Here's how the part is built. I have some questions about the finished solid (model axes, mm). Face numbers are marked on the shaded views. A direction names the side the tool comes from. Round coordinates to 2 decimals unless told otherwise and drop trailing zeros. Order: outer loops, then holes, each group sorted by start corner. A loop starts at its lowest first (then second) coordinate and runs counter-clockwise, first axis right, second up.
```python
from build123d import *

# Parameters (mm, degrees)
BOSS_EXTRUDE1_DEPTH        = 50
SKETCH2_W                  = 92
SKETCH2_H                  = 47.229685849
CUT_EXTRUDE4_DEPTH         = 152.455959439
CONVERT_SOLID1_START       = -117.963163746
CONVERT_SOLID1_DEPTH       = 125
CONVERT_SOLID1_2_DEPTH     = 125
FILLET1_R                  = 2
FILLET2_R                  = 75
F_6_5_6_5_DIAMETER_HOLE1_D = 6.5
F_6_5_6_5_DIAMETER_HOLE2_D = 6.5


# Read off the part's stored shape, not the designer's step: Convert-Solid1
with BuildPart() as part:
    # Sketch1 → Boss-Extrude1 (new, symmetric)
    with BuildSketch(Plane(origin=(0, 0, 0), x_dir=(0, 0, -1), z_dir=(1, 0, 0))):
        Polygon((-127.407338719, 17.525945159), (-7.036836254, 51.229685849), (0, 26.098127798), (0, 0), (-122.500074074, 0), align=None)
    extrude(amount=BOSS_EXTRUDE1_DEPTH, both=True)

    # Sketch2 → Cut-Extrude4 (cut, through all)
    with BuildSketch(Plane(origin=(0, 1.897341635, -6.776220126), x_dir=(-1, 0, 0), z_dir=(0, 0.2696299255199709, -0.9629640197141818))):
        with Locations((0, 23.614842925)):
            Rectangle(SKETCH2_W, SKETCH2_H)
    extrude(amount=-CUT_EXTRUDE4_DEPTH, mode=Mode.SUBTRACT)

    # Convert-Solid1 outline → Convert-Solid1 (cut)
    with BuildSketch(Plane(origin=(0, 0, 0), x_dir=(1, 0, 0), z_dir=(0, 0.26962992551997095, -0.9629640197141818)).offset(CONVERT_SOLID1_START)):
        with BuildLine():
            Line((50, -51.229685849), (50, -45.229685849))
            ThreePointArc((50, -45.229685849), (48.242640687, -49.472326536), (44, -51.229685849))
            Line((44, -51.229685849), (50, -51.229685849))
        make_face()
        with BuildLine():
            Line((-50, -51.229685849), (-44, -51.229685849))
            ThreePointArc((-44, -51.229685849), (-48.242640687, -49.472326536), (-50, -45.229685849))
            Line((-50, -45.229685849), (-50, -51.229685849))
        make_face()
    extrude(amount=CONVERT_SOLID1_DEPTH, mode=Mode.SUBTRACT)

    # Convert-Solid1 2 outline → Convert-Solid1 2 (add)
    with BuildSketch(Plane(origin=(0, 0, 0), x_dir=(1, 0, 0), z_dir=(0, 0.26962992551997095, -0.9629640197141818)).offset(CONVERT_SOLID1_START)):
        with BuildLine():
            Line((46, -47.229685849), (46, -45.229685849))
            ThreePointArc((46, -45.229685849), (45.414213562, -46.643899411), (44, -47.229685849))
            Line((44, -47.229685849), (46, -47.229685849))
        make_face()
        with BuildLine():
            Line((-46, -47.229685849), (-44, -47.229685849))
            ThreePointArc((-44, -47.229685849), (-45.414213562, -46.643899411), (-46, -45.229685849))
            Line((-46, -45.229685849), (-46, -47.229685849))
        make_face()
    extrude(amount=CONVERT_SOLID1_2_DEPTH)

    # Fillet1
    fillet1_edges = [part.edges().sort_by_distance(p)[0] for p in [
        (48, 0, 122.500074074),
        (48, 0, 0),
        (-48, 0, 0),
        (-48, 0, 122.500074074),
    ]]
    fillet(fillet1_edges, radius=FILLET1_R)

    # Fillet2
    fillet2_edges = [part.edges().sort_by_distance(p)[0] for p in [
        (48, 26.098127798, 0),
        (-48, 26.098127798, 0),
    ]]
    fillet(fillet2_edges, radius=FILLET2_R)

    # Ø6.5 (6.5) Diameter Hole1 (through all)
    with Locations(Plane(origin=(92.5, 101.400740105, -186.980648929), x_dir=(-1, 0, 0), z_dir=(0, -0.9629640197141818, -0.2696299255199709))):
        with Locations((92.5, -300.359475049), (92.5, -225.359475049), (-92.5, -300.359475049), (-92.5, -225.359475049)):
            Hole(F_6_5_6_5_DIAMETER_HOLE1_D / 2)

    # Ø6.5 (6.5) Diameter Hole2 (through all)
    with Locations(Plane(origin=(-92.5, 101.400740105, -186.980648929), x_dir=(-1, 0, 0), z_dir=(0, -0.9629640197141818, -0.2696299255199709))):
        with Locations((92.5, -300.359475049), (92.5, -225.359475049), (-92.5, -300.359475049), (-92.5, -225.359475049)):
            Hole(F_6_5_6_5_DIAMETER_HOLE2_D / 2)


solid = part.part
```
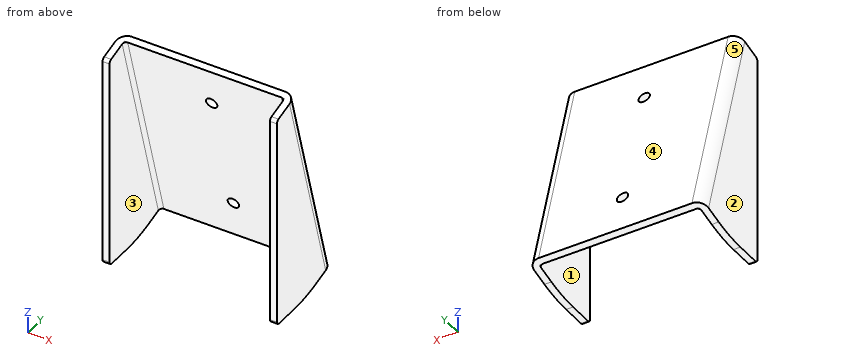
1) For the marked faces 1 and 2, which set-ups out of +Z, -Z, +X, -X, +Y, -Y let a thin tool reach every point of the face, with its end or its side?
2) I'm going to push flat-ended pins straight in: pin 1 (1 mm diameter, centred on x = 6.5, z = 34.5, fed in from +Y); pin 2 (10 mm diameter, centred on x = -33.5, z = 15.5, fed in from +Y); pin 3 (4 mm diameter, centred on y = 25, z = 105.5, fed in from -X). Where does each tip first touch, or does it pass through?
3) I need wall thicknesses on line 1 (X direction, y = 6.5, z = 26); line 2 (X direction, y = 27, z = 91); line 3 (Y direction, x = -42.5, z = 66). Which ranges of each line are inside material? Lowest first, please.
4) We'd pull the mould along X, two halves only. Please class the marked faces 3, 4 and 5: +X half, -X half, draft (parallel to the pull), parting line (faces both ways), or undercut.
5) If we section it at A-A (x = 22): Write out the boundary of the cut face in (y, z).
Solutions:
1. face 1: -Z, -Y
1. face 2: +Z, -Z, -X, +Y, -Y
2. pin 1: stops at y = 43.68
2. pin 2: stops at y = 50.26
2. pin 3: stops at x = -46.83
3. line 1: x = -50 to -46, 46 to 50
3. line 2: x = -46.8 to 46.8
3. line 3: y = 30.57 to 34.72
4. face 3: undercut
4. face 4: draft
4. face 5: -X half
5. outline: (13.67, 126.33) - (47.38, 5.96) - (51.23, 7.04) - (17.53, 127.41) - close
